The listing builds one solid part. Answer for the finished solid, in the listing's coordinates (mm). Coordinates: 2 decimals unless noted, no trailing zeros. Order: outer loops, then holes, each group sorted by start corner. A loop starts at its lowest first (then second) coordinate and runs counter-clockwise, first axis right, second up. Notation, with made-up numbers: (-6.75, -19.75) -> (44.25, -19.75) arc R8 cw to (44.25, -4.75) -> close; hole circle Ø7 at (5.5, -37.5). An arc over 180 degrees is marked (long way). Answer in a Markdown table with one row per item.
```python
from build123d import *

# Parameters (mm, degrees)
SKETCH1_R           = 2
SKETCH1_R_2         = 1.5
SKETCH1_W           = 20
SKETCH1_H           = 40
SKETCH1_W_2         = 4
SKETCH1_H_2         = 2
BOSS_EXTRUDE1_DEPTH = 2
BOSS_EXTRUDE2_DEPTH = 2
SKETCH4_R           = 1.5
CUT_EXTRUDE1_DEPTH  = 2


with BuildPart() as part:
    # Sketch1 → Boss-Extrude1 (new body)
    with BuildSketch(Plane(origin=(0, 0, 0), x_dir=(1, 0, 0), z_dir=(0, 1, 0))):
        Polygon((0, 0), (5, 0), (5, -2), (9, -2), (9, 0), (12.5, 0), (12.5, 2), (11.4, 2), (11.4, 4.3), (12.5, 4.3), (12.5, 6), (15.5, 6), (15.5, 4.3), (16.6, 4.3), (16.6, 2), (15.5, 2), (15.5, 0), (19, 0), (19, -2), (23, -2), (23, 0), (28, 0), (28, 66), (0, 66), align=None)
        with Locations(Location((18.75, 57.25, 0), (0, 0, 270))):
            Circle(SKETCH1_R, mode=Mode.SUBTRACT)
        with Locations(Location((9.25, 57.25, 0), (0, 0, 90))):
            Circle(SKETCH1_R, mode=Mode.SUBTRACT)
        with Locations(Location((18.75, 8.75, 0), (0, 0, 90))):
            Circle(SKETCH1_R, mode=Mode.SUBTRACT)
        with Locations(Location((9.25, 8.75, 0), (0, 0, 270))):
            Circle(SKETCH1_R, mode=Mode.SUBTRACT)
        with Locations(Location((14, 64, 0), (0, 0, 270))):
            Circle(SKETCH1_R_2, mode=Mode.SUBTRACT)
        with Locations((14, 33)):
            Rectangle(SKETCH1_W, SKETCH1_H, mode=Mode.SUBTRACT)
        with Locations((7, 64)):
            Rectangle(SKETCH1_W_2, SKETCH1_H_2, mode=Mode.SUBTRACT)
        with Locations((21, 64)):
            Rectangle(SKETCH1_W_2, SKETCH1_H_2, mode=Mode.SUBTRACT)
    extrude(amount=BOSS_EXTRUDE1_DEPTH)

    # Sketch2 → Boss-Extrude2 (add)
    with BuildSketch(Plane(origin=(0, 2, 0), x_dir=(1, 0, 0), z_dir=(0, 1, 0))):
        with BuildLine():
            Line((9, 186), (0, 66))
            Line((0, 66), (28, 66))
            Line((28, 66), (19, 186))
            ThreePointArc((19, 186), (14, 191), (9, 186))
        make_face()
    extrude(amount=-BOSS_EXTRUDE2_DEPTH)

    # Sketch4 → Cut-Extrude1 (cut)
    with BuildSketch(Plane(origin=(0, 2, 0), x_dir=(1, 0, 0), z_dir=(0, 1, 0))):
        with Locations(Location((14, 176, 0), (0, 0, 270))):
            Circle(SKETCH4_R)
        with BuildLine():
            Line((1.336247038, 176), (8.25, 176))
            ThreePointArc((8.25, 176), (14, 181.75), (19.75, 176))
            Line((19.75, 176), (26.690607085, 176))
            Line((26.690607085, 176), (26.690607085, 198.806068599))
            Line((26.690607085, 198.806068599), (1.336247038, 198.806068599))
            Line((1.336247038, 198.806068599), (1.336247038, 176))
        make_face()
    extrude(amount=-CUT_EXTRUDE1_DEPTH, mode=Mode.SUBTRACT)


solid = part.part
```
(1) A cutting plane is placed at B-B, the plane z = -8.75. Determine the outline of the cut face in (x, y), then the cut area to 3 significant figures.
Check values:
| item | result |
|---|---|
| outline | (0, 0) -> (7.25, 0) -> (7.25, 2) -> (0, 2) -> close; (11.25, 0) -> (16.75, 0) -> (16.75, 2) -> (11.25, 2) -> close; (20.75, 0) -> (28, 0) -> (28, 2) -> (20.75, 2) -> close |
| area | 40.0 mm² |
(2) Flat-ended cylindrical pins translate along their axes: pin 1 (1 mm diameter, centred on x = 17.5, y = 1, fed in from -Z); pin 2 (0.6 mm diameter, centred on x = 17, y = 1.5, fed in from +Z). Find the tip coordinate at first contact, or state that the pin passes through.
Check values:
| item | result |
|---|---|
| pin 1 | z = -180.91 |
| pin 2 | z = 0 |
(3) For a pull along Z with two mould halves and no side action, classify faces 1 (the cylindrical face through (11.233, 0.986, -9.01)), 2 (the flat face through (14, 2, -91)), 3 (the flat face through (4.215, 1.014, -122.205)) as released by +Z, released by -Z, zero draft, split by the parting line, or undercut.
Check values:
| item | result |
|---|---|
| face 1 | undercut |
| face 2 | zero draft |
| face 3 | released by -Z |
(4) Find the intervals of material crossed by line 1 along X through (y, z) = (0.65, -8.75); line 2 along X through (y, z) = (1.6, -64); line 3 along X through (y, z) = (0.8, -58), in increasing order. Write a range as from..to.
Check values:
| item | result |
|---|---|
| line 1 | 0..7.25, 11.25..16.75, 20.75..28 |
| line 2 | 0..5, 9..12.5, 15.5..19, 23..28 |
| line 3 | 0..7.4, 11.1..16.9, 20.6..28 |
(5) A cutting plane is placed at C-C, the plane y = 0.65. Count the separate pieces of the cut face and the enclosed holes in it, then the cut area to 3 significant figures.
Check values:
| item | result |
|---|---|
| separate pieces | 1 |
| enclosed holes | 9 |
| area | 3,180 mm² |
(6) A cutting plane is placed at D-D, the plane z = -170. Determine the outline of the cut face in (x, y), then the cut area to 3 significant figures.
Check values:
| item | result |
|---|---|
| outline | (7.8, 0) -> (20.2, 0) -> (20.2, 2) -> (7.8, 2) -> close |
| area | 24.8 mm² |
(7) A cutting plane is placed at A-A, the plane x = 14. Determine the outline of the cut face in (y, z), then the cut area to 4 significant figures.
Check values:
| item | result |
|---|---|
| outline | (0, -181.75) -> (2, -181.75) -> (2, -177.5) -> (0, -177.5) -> close; (0, -174.5) -> (2, -174.5) -> (2, -65.5) -> (0, -65.5) -> close; (0, -62.5) -> (2, -62.5) -> (2, -53) -> (0, -53) -> close; (0, -13) -> (2, -13) -> (2, -6) -> (0, -6) -> close |
| area | 259.5 mm² |
